from build123d import *

# Parameters (mm, degrees)
SKETCH1_W           = 53.594
SKETCH1_H           = 38.1
BOSS_EXTRUDE1_DEPTH = 42.5694094
CUT_EXTRUDE1_DEPTH  = 79.333144024
SKETCH5_W           = 25.654
SKETCH5_H           = 25.654
CUT_EXTRUDE2_DEPTH  = 79.333144024
SKETCH6_R           = 9.4107
BOSS_EXTRUDE2_DEPTH = 50.8


with BuildPart() as part:
    # Sketch1 → Boss-Extrude1 (new body)
    with BuildSketch(Plane(origin=(0, 0, 0), x_dir=(1, 0, 0), z_dir=(0, 1, 0))):
        with Locations((26.797, 19.05)):
            Rectangle(SKETCH1_W, SKETCH1_H)
    extrude(amount=BOSS_EXTRUDE1_DEPTH)

    # Sketch4 → Cut-Extrude1 (cut, through all)
    with BuildSketch(Plane.XY):
        Polygon((0, -5.737e-06), (15.494, 42.5694094), (0, 42.5694094), align=None)
    extrude(amount=-CUT_EXTRUDE1_DEPTH, mode=Mode.SUBTRACT)

    # Sketch5 → Cut-Extrude2 (cut, through all)
    with BuildSketch(Plane(origin=(0, 42.5694094, 0), x_dir=(1, 0, 0), z_dir=(0, 1, 0))):
        with Locations((34.544, 19.05)):
            Rectangle(SKETCH5_W, SKETCH5_H)
    extrude(amount=-CUT_EXTRUDE2_DEPTH, mode=Mode.SUBTRACT)


with BuildPart() as boss_extrude2_tool:
    # Sketch6 → Boss-Extrude2 (new body)
    with BuildSketch(Plane(origin=(0, 0, 0), x_dir=(0, 0, 1), z_dir=(-0.9396926207859096, 0.3420201433256656, 0))):
        with Locations(Location((-19.05, 22.650709993, 0), (0, 0, 90))):
            Circle(SKETCH6_R)
    extrude(amount=BOSS_EXTRUDE2_DEPTH)


with BuildPart() as part_1:
    add(part.part)


with BuildPart() as part_2:
    # Boss-Extrude2: joined with boss_extrude2_tool
    add(part_1.part.fuse(boss_extrude2_tool.part, tol=0.00001))


solid = part_2.part
CAD build for the part. Positions are in the model's coordinates, mm. A direction names the side the tool comes from. Round coordinates to 2 decimals unless told otherwise and drop trailing zeros. Write each loop counter-clockwise with the first axis right and the second up, starting at its lowest first coordinate (ties: lowest second). Pieces come first, ordered by that corner, then holes. Notation, with made-up numbers: M 68.5,-11.75 L 98.5,-11.75 A16 cw 98.5,18.25 Z; hole C 13,35.25 d9. An arc over 180 degrees is marked long. Put each result on its own line as item: value. Start each with the question number.
1) Pin check, flat tips, straight feed: pin 1 Ø6 at (x, y) = (-19, 35.5) entering from -Z; pin 2 Ø1.5 at (x, z) = (-24, -15.5) entering from +Y; pin 3 Ø19 at (x, z) = (26.5, -14) entering from +Y; pin 4 Ø8 at (x, z) = (23, -34) entering from -Y. Stop position of each tip, or through.
2) Saw through at B-B, the plane z = -8. Write the cut outline in (x, y), and give its area (3 significant figures).
3) Saw through at D-D, the plane z = -20. Write the cut outline in (x, y).
4) Saw through at A-A, the plane x = 39.5. Write the cut outline in (y, z), and give its area (3 significant figures).
5) Pull direction Y, two halves, no side cores. Call faces 1 (the flat face through (-40.034, 38.536, -19.182)), 2 (the flat face through (5.92, 16.26, -27.25)), 3 (the flat face through (20, 0, -19)), 4 (the flat face through (53.594, 21, -19)): pulls with the +Y half, pulls with the -Y half, needs draft (parallel to the pull), parting line crosses it, or undercut.
6) Drill centre lines: probe 1 along Z at (x, y) = (33.5, 20.5); probe 2 along Y at (x, z) = (47.5, -33); probe 3 along X at (y, z) = (7, -19). Where is each one in solid material? Low to high. Write a range as [from, to].
7) Saw through at C-C, the plane y = 10. Write the cut outline in (x, z).
8) 3-axis set-ups, long thin cutter, end or side, ignore diameter. For faces 5 (the flat face through (47.371, 22, -19)), 6 (the flat face through (32, 21, -38.1)): which of +Z, -Z, +X, -X, +Y, -Y reach the whole face in a straight line?
Resolved:
1. pin 1: z = -28.38
1. pin 2: y = 42.52
1. pin 3: y = 42.57
1. pin 4: y = 0
2. outline: M 0,0 L 21.72,0 L 21.72,42.57 L 15.49,42.57 Z; M 47.37,0 L 53.59,0 L 53.59,42.57 L 47.37,42.57 Z
2. area: 860 mm²
3. outline: M -43.19,29.86 L 4.54,12.49 L 0,0 L 21.72,0 L 21.72,42.57 L 15.49,42.57 L 10.95,30.08 L -36.79,47.46 Z; M 47.37,0 L 53.59,0 L 53.59,42.57 L 47.37,42.57 Z
4. outline: M 0,-38.1 L 42.57,-38.1 L 42.57,-31.88 L 0,-31.88 Z; M 0,-6.22 L 42.57,-6.22 L 42.57,0 L 0,0 Z
4. area: 530 mm²
5. face 1: pulls with the +Y half
5. face 2: undercut
5. face 3: pulls with the -Y half
5. face 4: needs draft
6. probe 1: [-38.1, -31.88], [-6.22, 0]
6. probe 2: [0, 42.57]
6. probe 3: [2.55, 21.72], [47.37, 53.59]
7. outline: M 3.64,-38.1 L 53.59,-38.1 L 53.59,0 L 3.64,0 Z; hole M 21.72,-31.88 L 47.37,-31.88 L 47.37,-6.22 L 21.72,-6.22 Z
8. face 5: +Y, -Y
8. face 6: -Z, +X, -X, +Y, -Y
